Can you work these out from the drawing? Everything is in mm from the part's minimum corner. A direction names the side the tool comes from. Coordinates: 2 decimals unless noted, no trailing zeros. Loops run counter-clockwise (first coordinate to the right, second up) from the corner with the lowest first, then second, coordinate; pieces in that order, holes last.
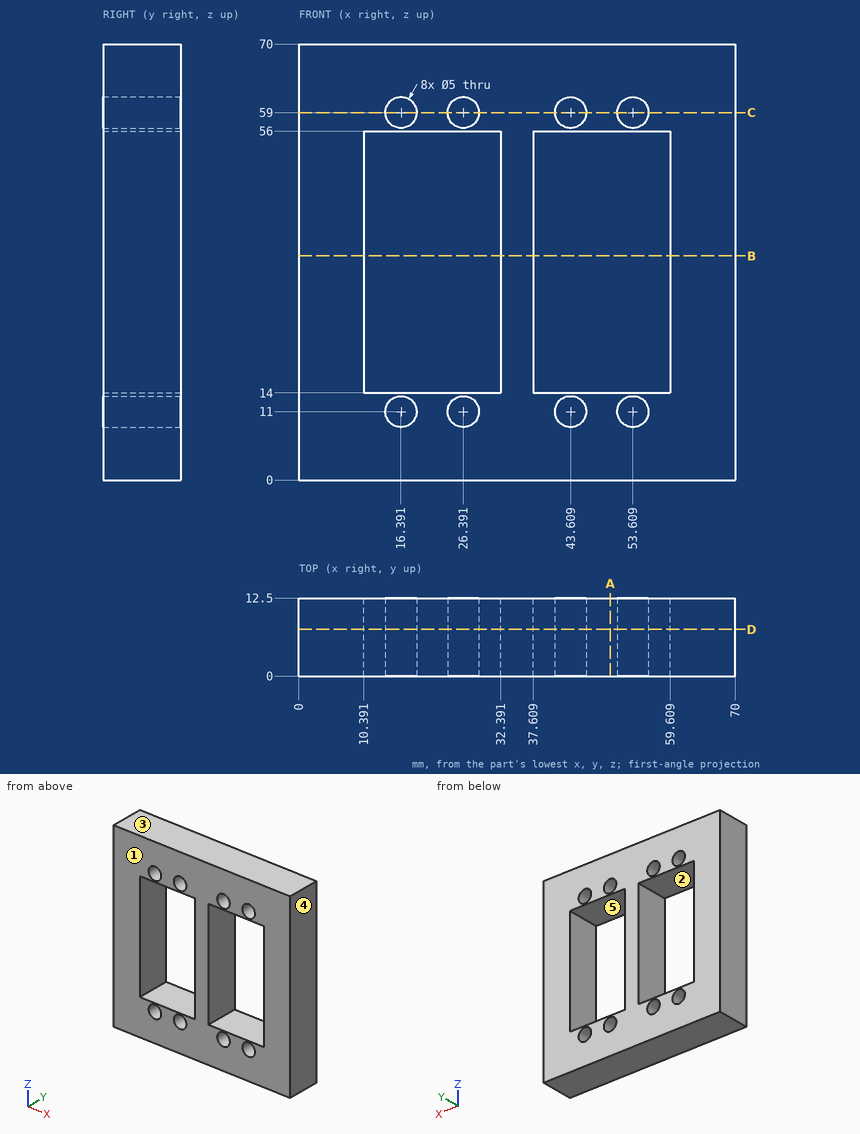
(1) Imagine slicing it at C-C, the plane z = 59. Write out the boundary of the cut face in (x, y), and give its area (3 significant figures).
Answers:
outline: (0, 0) - (13.89, 0) - (13.89, 12.5) - (0, 12.5) - close; (18.89, 0) - (23.89, 0) - (23.89, 12.5) - (18.89, 12.5) - close; (28.89, 0) - (41.11, 0) - (41.11, 12.5) - (28.89, 12.5) - close; (46.11, 0) - (51.11, 0) - (51.11, 12.5) - (46.11, 12.5) - close; (56.11, 0) - (70, 0) - (70, 12.5) - (56.11, 12.5) - close
area: 625 mm2
(2) Imagine slicing it at B-B, the plane z = 36. Write out the boundary of the cut face in (x, y), and give its area (3 significant figures).
Answers:
outline: (0, 0) - (10.39, 0) - (10.39, 12.5) - (0, 12.5) - close; (32.39, 0) - (37.61, 0) - (37.61, 12.5) - (32.39, 12.5) - close; (59.61, 0) - (70, 0) - (70, 12.5) - (59.61, 12.5) - close
area: 325 mm2
(3) Which directions (+Z, -Z, +X, -X, +Y, -Y) give clear straight access to the entire face, cutting with the end or side of a thin tool? Please do the marked faces 4 and 5.
Answers:
face 4: +Z, -Z, +X, +Y, -Y
face 5: +Y, -Y
(4) Imagine slicing it at D-D, the plane y = 7.5. State how many separate pieces and enclosed holes the cut face has.
Answers:
separate pieces: 1
enclosed holes: 10
(5) Imagine slicing it at A-A, the plane x = 50. Write out the boundary of the cut face in (y, z).
Answers:
outline: (0, 0) - (12.5, 0) - (12.5, 14) - (0, 14) - close; (0, 56) - (12.5, 56) - (12.5, 70) - (0, 70) - close
(6) I need wall thicknesses on probe 1 along X at (y, z) = (8.75, 59); probe 2 along X at (y, z) = (3.75, 31.5); probe 3 along Z at (x, y) = (29, 5.75). Which ranges of each line are inside material? Lowest first, please.
Answers:
probe 1: x = 0 to 13.89, 18.89 to 23.89, 28.89 to 41.11, 46.11 to 51.11, 56.11 to 70
probe 2: x = 0 to 10.39, 32.39 to 37.61, 59.61 to 70
probe 3: z = 0 to 14, 56 to 70
(7) We'd pull the mould along Z, two halves only. Please class the marked faces 1, 2 and 3: +Z half, -Z half, draft (parallel to the pull), parting line (faces both ways), or undercut.
Answers:
face 1: draft
face 2: undercut
face 3: +Z half
